```python
from build123d import *

# Parameters (mm, degrees)
ESQUISSE1_W             = 329
ESQUISSE1_H             = 150
BOSS_EXTRU_1_DEPTH      = 370
ESQUISSE2_W             = 319
ESQUISSE2_H             = 335
ENL_V_MAT_EXTRU_1_DEPTH = 90
ESQUISSE3_W             = 209
ESQUISSE3_H             = 10.713791462
ENL_V_MAT_EXTRU_2_DEPTH = 30
ESQUISSE4_W             = 208.8
ESQUISSE4_H             = 8.713791462
ENL_V_MAT_EXTRU_3_DEPTH = 30
ESQUISSE6_W             = 90.150575604
ESQUISSE6_H             = 11.402147775
BOSS_EXTRU_3_DEPTH      = 30
ESQUISSE7_W             = 5
ESQUISSE7_H             = 90
BOSS_EXTRU_4_DEPTH      = 329
ESQUISSE8_W             = 5
ESQUISSE8_H             = 92.498011514
BOSS_EXTRU_5_DEPTH      = 329
ESQUISSE9_W             = 5
ESQUISSE9_H             = 90
BOSS_EXTRU_6_DEPTH      = 329
ESQUISSE10_W            = 5
ESQUISSE10_H            = 90
BOSS_EXTRU_7_DEPTH      = 329
ESQUISSE11_W            = 5
ESQUISSE11_H            = 91.858335329
BOSS_EXTRU_8_DEPTH      = 329


with BuildPart() as part:
    # Esquisse1 → Boss.-Extru.1 (new body)
    with BuildSketch(Plane.XY):
        with Locations((55.821656051, -51.75955414)):
            Rectangle(ESQUISSE1_W, ESQUISSE1_H)
    extrude(amount=BOSS_EXTRU_1_DEPTH)

    # Esquisse2 → Enlèv. mat.-Extru.1 (cut)
    with BuildSketch(Plane(origin=(0, 23.24044586, 0), x_dir=(1, 0, 0), z_dir=(0, 1, 0))):
        with Locations((55.821656051, -197.5)):
            Rectangle(ESQUISSE2_W, ESQUISSE2_H)
    extrude(amount=-ENL_V_MAT_EXTRU_1_DEPTH, mode=Mode.SUBTRACT)

    # Esquisse3 → Enlèv. mat.-Extru.2 (cut)
    with BuildSketch(Plane(origin=(0, -126.75955414, 0), x_dir=(-1, 0, 0), z_dir=(0, -1, 0))):
        with Locations((-55.821656051, -5.356895731)):
            Rectangle(ESQUISSE3_W, ESQUISSE3_H)
    extrude(amount=-ENL_V_MAT_EXTRU_2_DEPTH, mode=Mode.SUBTRACT)

    # Esquisse4 → Enlèv. mat.-Extru.3 (cut)
    with BuildSketch(Plane(origin=(0, -96.75955414, 0), x_dir=(-1, 0, 0), z_dir=(0, -1, 0))):
        with Locations((-55.821656051, -6.356895731)):
            Rectangle(ESQUISSE4_W, ESQUISSE4_H)
    extrude(amount=-ENL_V_MAT_EXTRU_3_DEPTH, mode=Mode.SUBTRACT)

    # Esquisse6 → Boss.-Extru.3 (add)
    with BuildSketch(Plane(origin=(0, -66.75955414, 0), x_dir=(-1, 0, 0), z_dir=(0, -1, 0))):
        with Locations((3.603056147, -11.057969619)):
            Rectangle(ESQUISSE6_W, ESQUISSE6_H)
    extrude(amount=-BOSS_EXTRU_3_DEPTH)

    # Esquisse7 → Boss.-Extru.4 (add)
    with BuildSketch(Plane.ZY.offset(108.678343949)):
        with Locations((86.839910946, -21.75955414)):
            Rectangle(ESQUISSE7_W, ESQUISSE7_H)
    extrude(amount=-BOSS_EXTRU_4_DEPTH)

    # Esquisse8 → Boss.-Extru.5 (add)
    with BuildSketch(Plane.ZY.offset(108.678343949)):
        with Locations((146.839910946, -23.008559897)):
            Rectangle(ESQUISSE8_W, ESQUISSE8_H)
    extrude(amount=-BOSS_EXTRU_5_DEPTH)

    # Esquisse9 → Boss.-Extru.6 (add)
    with BuildSketch(Plane.ZY.offset(108.678343949)):
        with Locations((206.839910946, -21.75955414)):
            Rectangle(ESQUISSE9_W, ESQUISSE9_H)
    extrude(amount=-BOSS_EXTRU_6_DEPTH)

    # Esquisse10 → Boss.-Extru.7 (add)
    with BuildSketch(Plane.ZY.offset(108.678343949)):
        with Locations((266.839910946, -21.75955414)):
            Rectangle(ESQUISSE10_W, ESQUISSE10_H)
    extrude(amount=-BOSS_EXTRU_7_DEPTH)

    # Esquisse11 → Boss.-Extru.8 (add)
    with BuildSketch(Plane.ZY.offset(108.678343949)):
        with Locations((326.839910946, -22.688721805)):
            Rectangle(ESQUISSE11_W, ESQUISSE11_H)
    extrude(amount=-BOSS_EXTRU_8_DEPTH)


solid = part.part
```
The listing builds one solid part. Answer for the finished solid, in the listing's coordinates (mm). A direction names the side the tool comes from. Give positions to 0.01 mm unless a question says otherwise; leave off trailing zeros. Order: outer loops, then holes, each group sorted by start corner. A loop starts at its lowest first (then second) coordinate and runs counter-clockwise, first axis right, second up. Notation, with made-up numbers: (39, 17.5) -> (68, 17.5) arc R15 cw to (68, 27.5) -> close; hole circle Ø1 at (34.5, 46). An arc over 180 degrees is marked (long way). One line per item, written item: value.
1) Find the intervals of material crossed by line 1 (Z direction, x = 90.5, y = -77.5); line 2 (X direction, y = -10, z = 76.5); line 3 (Y direction, x = 1.5, z = 83), in increasing order.
Reported:
line 1: z = 0 to 2, 10.71 to 370
line 2: x = -108.68 to -103.68, 215.32 to 220.32
line 3: y = -126.76 to -66.76
2) Determine the mould class of faces 1 (the flat face through (-48.678, -112, 5)), 2 (the flat face through (-103.678, -21, 237)) for opening direction Z: pulls with the +Z half, pulls with the -Z half, needs draft (parallel to the pull), parting line crosses it, or undercut.
Reported:
face 1: needs draft
face 2: undercut
3) Flat-ended cylindrical pins translate along their axes: P1, Ø1.5, axis at x = -35.5, z = 290, coming from the +Y side; P2, Ø7, axis at x = 91.5, z = 7, coming from the -Y side; P3, Ø8.5, axis at x = 92, z = 6, coming from the -Y side. Find the tip coordinate at first contact, or state that the pin passes through.
Reported:
P1: stops at y = -66.76
P2: stops at y = -66.76
P3: stops at y = -96.76
4) Find section A-A, the plane y = -5.5. Determine the outline of the cut face in (x, z), plus the area to 3 significant figures.
Reported:
outline: (-108.68, 0) -> (220.32, 0) -> (220.32, 370) -> (-108.68, 370) -> close; hole (-103.68, 30) -> (215.32, 30) -> (215.32, 84.34) -> (-103.68, 84.34) -> close; hole (-103.68, 89.34) -> (215.32, 89.34) -> (215.32, 144.34) -> (-103.68, 144.34) -> close; hole (-103.68, 149.34) -> (215.32, 149.34) -> (215.32, 204.34) -> (-103.68, 204.34) -> close; hole (-103.68, 209.34) -> (215.32, 209.34) -> (215.32, 264.34) -> (-103.68, 264.34) -> close; hole (-103.68, 269.34) -> (215.32, 269.34) -> (215.32, 324.34) -> (-103.68, 324.34) -> close; hole (-103.68, 329.34) -> (215.32, 329.34) -> (215.32, 365) -> (-103.68, 365) -> close
area: 22,800 mm^2
5) Find section D-D, the plane y = -109.5. Determine the outline of the cut face in (x, z), plus the area to 3 significant figures.
Reported:
outline: (-108.68, 0) -> (-48.68, 0) -> (-48.68, 10.71) -> (160.32, 10.71) -> (160.32, 0) -> (220.32, 0) -> (220.32, 370) -> (-108.68, 370) -> close
area: 119,000 mm^2
6) Find section B-B, the plane z = 134. Determine the outline of the cut face in (x, y).
Reported:
outline: (-108.68, -126.76) -> (220.32, -126.76) -> (220.32, 23.24) -> (215.32, 23.24) -> (215.32, -66.76) -> (-103.68, -66.76) -> (-103.68, 23.24) -> (-108.68, 23.24) -> close
7) A tool of negligible diameter and unlimited length cuts with its end or side. For faces 3 (the flat face through (57, -66.76, 6)), 4 (the flat face through (220.322, -53, 182)), 5 (the flat face through (-103.678, -21, 297)), from which of +Z, -Z, +X, -X, +Y, -Y can it reach the whole face along a straight path? Write none if from no direction.
Reported:
face 3: -Y
face 4: +Z, -Z, +X, +Y, -Y
face 5: +Y
